```python
from build123d import *

# Parameters (mm, degrees)
F0_W     = 406.4
F0_H     = 609.6
F1_DEPTH = 609.6
F1_TAPER = 2
F2_W     = 203.2
F2_H     = 1930.4
F3_DEPTH = 152.4
F5_DEPTH = 304.8


with BuildPart() as f1:
    # F0 (on Top) → F1 (new body)
    with BuildSketch(Plane.XY):
        with Locations((203.2, 304.8)):
            Rectangle(F0_W, F0_H)
    extrude(amount=F1_DEPTH, taper=F1_TAPER)

    # F2 (on face) → F3 (join)
    with BuildSketch(Plane.XY.offset(609.6)):
        with Locations((283.5122989178, 304.8)):
            Rectangle(F2_W, F2_H)
    extrude(amount=F3_DEPTH)

    # F4 (on face) → F5 (join)
    with BuildSketch(Plane.XY.offset(609.6)):
        Polygon((181.9122989178, -152.4), (181.9122989178, 762), (131.1122989178, 762), (131.1122989178, 533.4), (-122.8877010822, 533.4), (-122.8877010822, 76.2), (131.1122989178, 76.2), (131.1122989178, -152.4), align=None)
    extrude(amount=F5_DEPTH)


solid = f1.part
```
Check sheet for the modelled part. Datum: model origin and axes. Units: mm. A direction names the side the tool comes from. Give positions to 0.01 mm unless a question says otherwise; leave off trailing zeros. Write each loop counter-clockwise with the first axis right and the second up, starting at its lowest first coordinate (ties: lowest second). Pieces come first, ordered by that corner, then holes.
Item 1: Cross-section at C-C (y = 460.5). Enter the section's corners in (x, z), and give its area (3 significant figures).
Item 2: Scan lines: L1, parallel to Z at x = 245, y = 402; L2, parallel to X at y = -554, z = 661.5; L3, parallel to Z at x = 312, y = -307.5. Record each from-to range of solid material in increasing order.
Item 3: Gauge pin test, flat ends, axial feed: pin 1 (10 mm diameter, centred on x = 25.5, z = 373, fed in from +Y); pin 2 (16.5 mm diameter, centred on x = 88, y = 566.5, fed in from +Z); pin 3 (8 mm diameter, centred on x = 178.5, z = 278, fed in from -Y); pin 4 (5 mm diameter, centred on x = 28.5, y = 412, fed in from -Z). Record the tip position at first contact, or that the pin passes through.
Item 4: Cross-section at B-B (x = 302). Enter the section's corners in (y, z).
Item 5: Cross-section at A-A (z = 694). Enter the section's corners in (x, y).
Item 6: Cross-section at D-D (x = 63.5). Enter the section's corners in (y, z).
Item 7: Access from +Z, -Z, +X, -X, +Y, -Y to the whole of each face (thin tool, end or side, straight path). Record for faces 1 (the face through (75, 561, 609.6)), 2 (the face through (2, 76.2, 760)), 3 (the face through (157, 762, 760)), 4 (the face through (181.912, -410, 685)), 5 (the face through (282, 318, 762)).
Report:
1. outline: (-122.89, 609.6) - (21.29, 609.6) - (0, 0) - (406.4, 0) - (385.11, 609.6) - (385.11, 762) - (181.91, 762) - (181.91, 914.4) - (-122.89, 914.4) - close
1. area: 359,000 mm2
2. L1: z = 0 to 762
2. L2: x = 181.91 to 385.11
2. L3: z = 609.6 to 762
3. pin 1: stops at y = 596.75
3. pin 2: stops at z = 609.6
3. pin 3: stops at y = 9.57
3. pin 4: stops at z = 0
4. outline: (-660.4, 609.6) - (21.29, 609.6) - (0, 0) - (609.6, 0) - (588.31, 609.6) - (1270, 609.6) - (1270, 762) - (-660.4, 762) - close
5. outline: (-122.89, 76.2) - (131.11, 76.2) - (131.11, -152.4) - (181.91, -152.4) - (181.91, -660.4) - (385.11, -660.4) - (385.11, 1270) - (181.91, 1270) - (181.91, 762) - (131.11, 762) - (131.11, 533.4) - (-122.89, 533.4) - close
6. outline: (0, 0) - (609.6, 0) - (588.31, 609.6) - (533.4, 609.6) - (533.4, 914.4) - (76.2, 914.4) - (76.2, 609.6) - (21.29, 609.6) - close
7. face 1: +Z, -X, +Y
7. face 2: +Z, -X, -Y
7. face 3: +Z, -Z, -X, +Y
7. face 4: +Z, -Z, -X, -Y
7. face 5: +Z, +X, +Y, -Y
